Verification items for this drawing (mm, ordinates from the low corner). Coordinates: 2 decimals unless noted, no trailing zeros. Write each loop counter-clockwise with the first axis right and the second up, starting at its lowest first coordinate (ties: lowest second). Pieces come first, ordered by that corner, then holes.
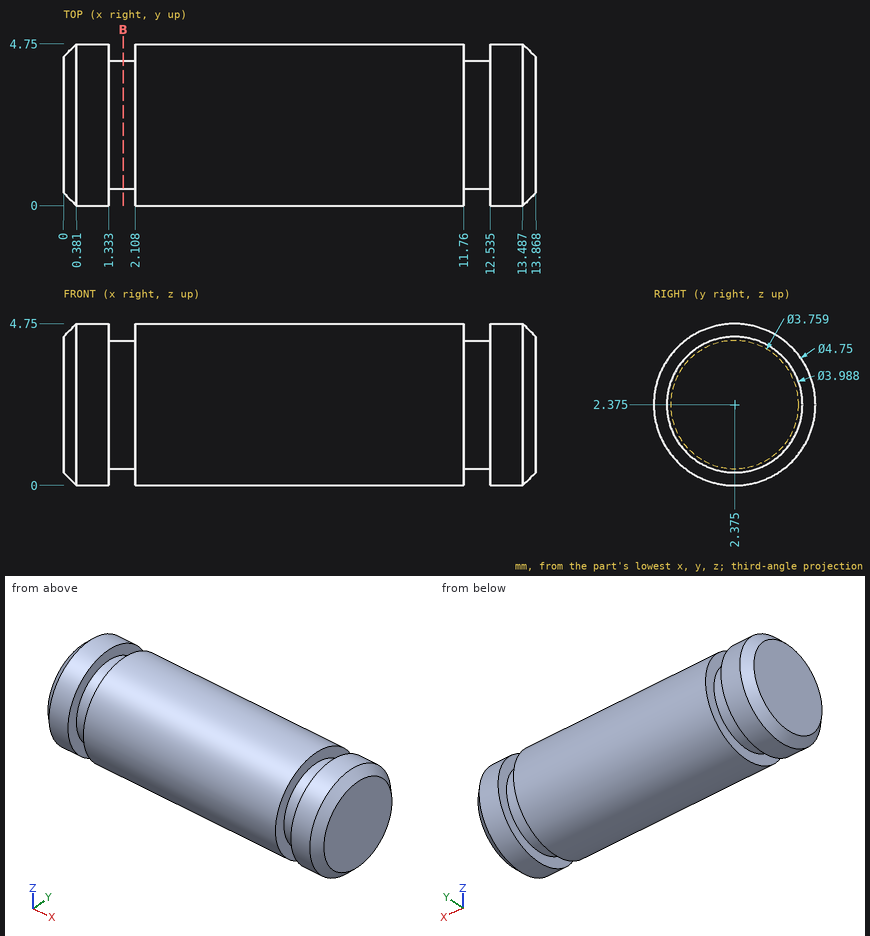
1. Thickness scan on line 1 along X through (y, z) = (2, 0.45) (1 decimal); line 2 along X through (y, z) = (0.5, 3.6) (1 decimal); line 3 along Y through (x, z) = (8.5, 3.65). Record the ranges inside material, lowest first.
Computed values:
line 1: x = 0 to 1.3, 2.1 to 11.8, 12.5 to 13.9
line 2: x = 0.2 to 1.3, 2.1 to 11.8, 12.5 to 13.6
line 3: y = 0.37 to 4.38
2. Gauge pin test, flat ends, axial feed: pin 1 Ø1 at (x, y) = (12.5, 1.5) entering from +Z; pin 2 Ø1.5 at (x, y) = (3.5, 4) entering from +Z. Record the tip position at first contact, or that the pin passes through.
Computed values:
pin 1: stops at z = 4.72
pin 2: stops at z = 4.58
3. Sectioned sample at B-B, the plane x = 1.75. Record the boundary of the cut face in (y, z) (1 decimal).
Computed values:
outline: circle Ø3.8 at (2.4, 2.4)
